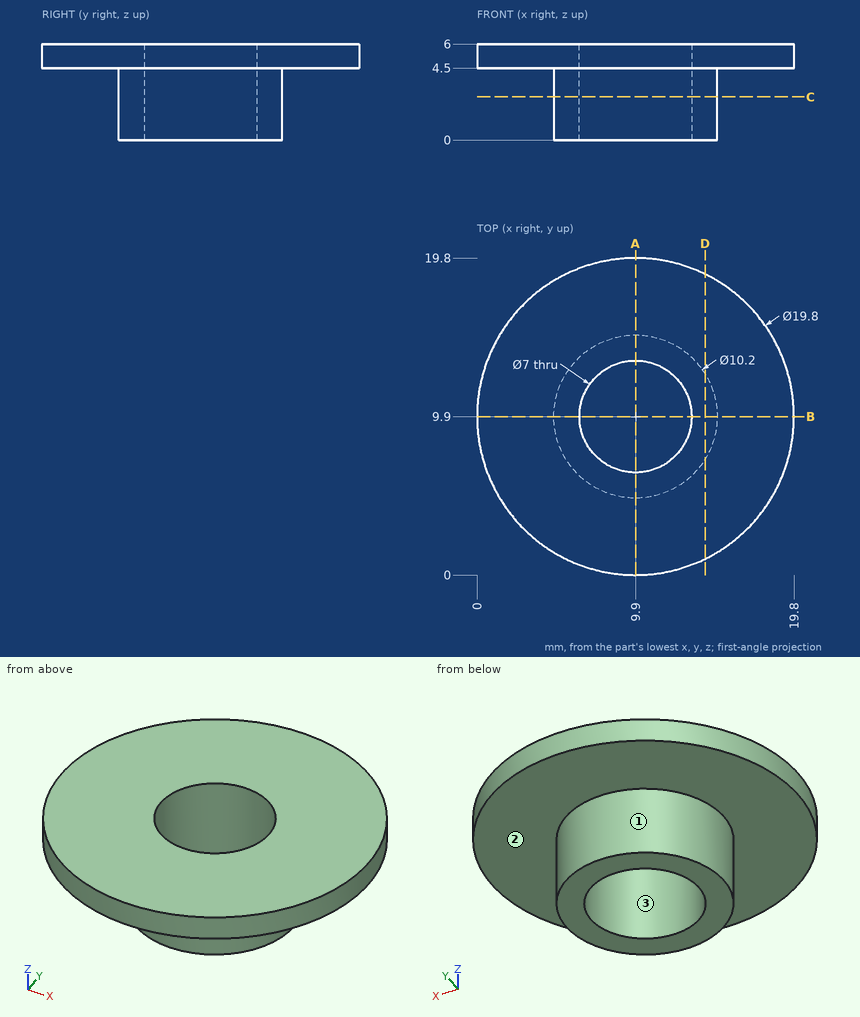
Job drawing, mm, ordinate dimensions from the low corner. One solid piece. Coordinates: 2 decimals unless noted, no trailing zeros. Write each loop counter-clockwise with the first axis right and the second up, starting at its lowest first coordinate (ties: lowest second). Pieces come first, ordered by that corner, then holes. Notation, with made-up numbers: (-26, -33.75) -> (31, -33.75) arc R6 ccw to (31, -29.75) -> close; hole circle Ø11 at (15, 71). An arc over 180 degrees is marked (long way). Use CSV: the item, a comma, the result in double quotes. Start each with the question number.
Item 1: Band-saw the part on A-A, the plane x = 9.9. Write the cut outline in (y, z), plus the area to 3 significant figures.
Item 2: Band-saw the part on D-D, the plane x = 14.25. Write the cut outline in (y, z), plus the area to 3 significant figures.
Item 3: Band-saw the part on C-C, the plane z = 2.7. Write the cut outline in (x, y), plus the area to 3 significant figures.
Item 4: Two-plate mould, pull along X, no slides. Class the marked faces 1, 2 and 3: +X half, -X half, draft (parallel to the pull), parting line (faces both ways), or undercut.
Item 5: Wall check: probe 1 along Y at (x, z) = (9.9, 1.75); probe 2 along Z at (x, y) = (13.75, 4); probe 3 along Y at (x, z) = (9.9, 4.85). Give the ranges that are in metal, low to high.
Response values:
1,outline,"(0, 4.5) -> (4.8, 4.5) -> (4.8, 0) -> (6.4, 0) -> (6.4, 6) -> (0, 6) -> close; (13.4, 0) -> (15, 0) -> (15, 4.5) -> (19.8, 4.5) -> (19.8, 6) -> (13.4, 6) -> close"
1,area,"33.6 mm2"
2,outline,"(1.01, 4.5) -> (7.24, 4.5) -> (7.24, 0) -> (12.56, 0) -> (12.56, 4.5) -> (18.79, 4.5) -> (18.79, 6) -> (1.01, 6) -> close"
2,area,"50.6 mm2"
3,outline,"circle Ø10.2 at (9.9, 9.9); hole circle Ø7 at (9.9, 9.9)"
3,area,"43.2 mm2"
4,face 1,"parting line"
4,face 2,"draft"
4,face 3,"undercut"
5,probe 1,"y = 4.8 to 6.4, 13.4 to 15"
5,probe 2,"z = 4.5 to 6"
5,probe 3,"y = 0 to 6.4, 13.4 to 19.8"
